```python
from build123d import *

# Parameters (mm, degrees)
F0_W     = 25.4
F0_H     = 304.8
F1_DEPTH = 25.4
F2_W     = 19.05
F2_H     = 19.05
F3_DEPTH = 304.8
F5_D     = 5.1054
F5_DEPTH = 25.4
F7_D     = 5.1054
F7_DEPTH = 25.4


with BuildPart() as f1:
    # F0 (on Right) → F1 (new body)
    with BuildSketch(Plane.YZ):
        with Locations((-14.18734, 160.249631)):
            Rectangle(F0_W, F0_H)
    extrude(amount=F1_DEPTH)

    # F2 (on face) → F3 (cut)
    with BuildSketch(Plane.XY.offset(312.649631)):
        with Locations((12.7, -14.18734)):
            Rectangle(F2_W, F2_H)
    extrude(amount=-F3_DEPTH, mode=Mode.SUBTRACT)

    # F5
    with Locations(Plane.YZ.offset(25.4)):
        with Locations((-14.18734, 20.549631), (-14.18734, 96.749631), (-14.18734, 122.149631), (-14.18734, 147.549631), (-14.18734, 45.949631), (-14.18734, 71.349631), (-14.18734, 172.949631), (-14.18734, 299.949631), (-14.18734, 198.349631), (-14.18734, 223.749631), (-14.18734, 249.149631), (-14.18734, 274.549631), (11.21266, 299.949631)):
            Hole(F5_D / 2, depth=F5_DEPTH)

    # F7
    with Locations(Plane(origin=(0, -1.48734, 0), x_dir=(-1, 0, 0), z_dir=(0, 1, 0))):
        with Locations((-12.7, 20.549631), (-12.7, 71.349631), (-12.7, 45.949631), (-12.7, 299.949631), (-12.7, 249.149631), (-12.7, 274.549631), (-12.7, 122.149631), (-12.7, 96.749631), (-12.7, 172.949631), (-12.7, 147.549631), (-12.7, 223.749631), (-12.7, 198.349631)):
            Hole(F7_D / 2, depth=F7_DEPTH)


solid = f1.part
```
Read the model definition and answer for the solid it produces. Units are mm, in the model's axes. Coordinates: 2 decimals unless noted, no trailing zeros. Write each loop counter-clockwise with the first axis right and the second up, starting at its lowest first coordinate (ties: lowest second). Pieces come first, ordered by that corner, then holes. Notation, with made-up numbers: (-9, -26.5) - (47, -26.5) arc R23 cw to (47, 5.5) - close; hole circle Ø11 at (67.25, 65). An arc over 180 degrees is marked (long way). Answer as a JSON object with one key per item and string values. Group by question number.
1. Consider L1, parallel to Y at x = 9, z = 175.5; L2, parallel to X at y = -22, z = 47 (3 decimals). Determine where each line is inside the solid, lowest interval first. Write a range as [from, to].
2. A cutting plane is placed at B-B (z = 54). Determine the outline of the cut face in (x, y) (3 decimals), plus the area to 3 significant figures.
3. A cutting plane is placed at A-A (x = 18.5). Determine the outline of the cut face in (y, z), plus the area to 3 significant figures.
4. The mould has two halves that part along X. Classify faces 1 (the cylindrical face through (13.878, -3.097, 119.885)), 2 (the cylindrical face through (23.79, -13.63, 170.46)): +X half, -X half, draft (parallel to the pull), parting line (faces both ways), or undercut.
Worked out:
{
 "1": {"L1": "y = [-26.89, -23.71], [-4.66, -1.49]", "L2": "x = [0, 3.175], [22.225, 25.4]"},
 "2": {"outline": "(0, -26.887) - (25.4, -26.887) - (25.4, -1.487) - (0, -1.487) - close; hole (3.175, -23.712) - (22.225, -23.712) - (22.225, -4.662) - (3.175, -4.662) - close", "area": "282 mm²"},
 "3": {"outline": "(-26.89, 7.85) - (-23.71, 7.85) - (-23.71, 312.65) - (-26.89, 312.65) - close; (-4.66, 7.85) - (-1.49, 7.85) - (-1.49, 312.65) - (-4.66, 312.65) - close", "area": "1,940 mm²"},
 "4": {"face 1": "undercut", "face 2": "draft"}
}
